```python
from build123d import *

# Parameters (mm, degrees)
F2_R     = 2.9933814251
F4_R     = 5.9933814251
F5_DEPTH = 5


# Not quite as in the source:
# - a fillet or chamfer that OpenCascade refuses, or shapes differently, is made with other operations: its cross-section is extruded or revolved along the edge and cut away or added


with BuildPart() as f3:
    # F3: sweep along a path in F0
    with BuildLine(Plane.XZ) as f3_path:
        Line((51.9430634924, -22.1786051989), (51.9430634924, 95.8719234608))
        ThreePointArc((51.9430634924, 95.8719234608), (46.1700643013, 104.9346197572), (35.5165706601, 103.533528376))
        Line((35.5165706601, 103.533528376), (-30.1489816492, 48.4537890892))
        ThreePointArc((-30.1489816492, 48.4537890892), (-33.11972376, 37.3728311031), (-23.7224888169, 30.7921841741))
        Line((-23.7224888169, 30.7921841741), (9.4017067552, 30.7921841741))
        ThreePointArc((9.4017067552, 30.7921841741), (16.472774567, 27.8632519859), (19.4017067552, 20.7921841741))
        Line((19.4017067552, 20.7921841741), (19.4017067552, -22.1786051989))
    # F2 (on line) → F3 (sweep)
    with BuildSketch(Plane.XY.offset(-22.1786051989)):
        with Locations((52.0414784551, 0)):
            Circle(F2_R)
    sweep(path=f3_path.line)

    # F4 (on line) → F5 (join)
    with BuildSketch(Plane.XY.offset(-22.1786051989)):
        with Locations((52.0414784551, 0)):
            Circle(F4_R)
        with Locations((19.3032917925, 0)):
            Circle(F4_R)
    extrude(amount=F5_DEPTH)

    # F6: fillet of radius 5 on 2 edges, made by hand

    # F6_s1 → F6_t2 (revolve, cut)
    with BuildSketch(Plane.XZ):
        with BuildLine():
            ThreePointArc((58.0348598802, -21.7611808938), (57.2181600129, -19.0225681063), (55.0348598802, -17.1786051989))
            Line((55.0348598802, -17.1786051989), (58.0348598802, -17.1786051989))
            Line((58.0348598802, -17.1786051989), (58.0348598802, -21.7611808938))
        make_face()
    revolve(axis=Axis((52.0414784551, 0, -17.1786051989), (0, 0, 1)), mode=Mode.SUBTRACT)

    # F6_s3 → F6_t4 (revolve, cut)
    with BuildSketch(Plane.XZ):
        with BuildLine():
            ThreePointArc((22.2966732176, -17.1786051989), (24.4799733503, -19.0225681063), (25.2966732176, -21.7611808938))
            Line((25.2966732176, -21.7611808938), (25.2966732176, -17.1786051989))
            Line((25.2966732176, -17.1786051989), (22.2966732176, -17.1786051989))
        make_face()
    revolve(axis=Axis((19.3032917925, 0, -17.1786051989), (0, 0, 1)), mode=Mode.SUBTRACT)


solid = f3.part
```
Read the model definition and answer for the solid it produces. Units are mm, in the model's axes. A direction names the side the tool comes from. Round coordinates to 2 decimals unless told otherwise and drop trailing zeros. One line per item, written item: value.
1) For faces 1 (the face through (25.02, 1.8, -21.97)), 2 (the face through (52, 0, -22.179)), 3 (the face through (49.05, 0.13, 40.14)), determine the directions among +Z, -Z, +X, -X, +Y, -Y from which every point of the face is accessible in a straight line to the end or side of a thin tool.
Answer list:
face 1: -Z
face 2: -Z, +X, -X, +Y, -Y
face 3: none
2) The mould has two halves that part along X. Classify faces 4 (the face through (19, 0, -22.179)), 5 (the face through (4.08, 0.13, 73.39)): pulls with the +X half, pulls with the -X half, needs draft (parallel to the pull), parting line crosses it, or undercut.
Answer list:
face 4: needs draft
face 5: undercut
3) Flat-ended cylindrical pins translate along their axes: P1, Ø1.5, axis at y = 4.5, z = 37.5, coming from the +X side; P2, Ø8, axis at x = 4.5, z = 73.5, coming from the +Y side; P3, Ø3, axis at y = -0.5, z = 59.5, coming from the +X side; P4, Ø4, axis at x = -27, y = 1, coming from the +Z side. Find the tip coordinate at first contact, or state that the pin passes through.
Answer list:
P1: passes through
P2: stops at y = 2.99
P3: stops at x = 55.03
P4: stops at z = 56.7
4) Consider L1, parallel to X at y = -2, z = -12; L2, parallel to Z at x = -6, y = 1.75; L3, parallel to Z at x = -24, y = 1.5. Determine where each line is inside the solid, lowest interval first. Write a range as [from, to].
Answer list:
L1: x = [17.08, 21.53], [49.81, 54.27]
L2: z = [28.27, 33.12], [65.67, 72.01]
L3: z = [28.11, 33.29], [50.36, 57.12]
